```python
from build123d import *

# Parameters (mm, degrees)
F1_DEPTH = 19.05
F2_W     = 6.35
F2_H     = 28.8036865525
F3_DEPTH = 25.4
F4_R     = 5.08
F6_D     = 5.1054


# Not quite as in the source:
# - a feature names something its author has since deleted; it is built from what else it names


with BuildPart() as f1:
    # F0 (on Front) → F1 (new body, symmetric)
    with BuildSketch(Plane.XZ):
        with BuildLine():
            Line((-63.5, 3.175), (-63.5, -3.175))
            Line((-63.5, -3.175), (-25.8909725642, -3.175))
            ThreePointArc((-25.8909725642, -3.175), (-21.6829722848, -1.5805476707), (-19.5881864455, 2.4020917642))
            ThreePointArc((-19.5881864455, 2.4020917642), (0, 19.7349206501), (19.5881864455, 2.4020917642))
            ThreePointArc((19.5881864455, 2.4020917642), (21.6829722848, -1.5805476707), (25.8909725642, -3.175))
            Line((25.8909725642, -3.175), (63.5, -3.175))
            Line((63.5, -3.175), (66.675, -3.175))
            ThreePointArc((66.675, -3.175), (68.9200640303, -2.2450640303), (69.85, 0))
            Line((69.85, 0), (69.85, 27.0641443402))
            ThreePointArc((69.85, 27.0641443402), (70.3149679849, 28.1866763553), (71.4375, 28.6516443402))
            Line((71.4375, 28.6516443402), (87.1900793672, 28.6516443402))
            Line((87.1900793672, 28.6516443402), (87.1900793672, 35.0016443402))
            Line((87.1900793672, 35.0016443402), (66.675, 35.0016443402))
            ThreePointArc((66.675, 35.0016443402), (64.4299359697, 34.0717083704), (63.5, 31.8266443402))
            Line((63.5, 31.8266443402), (63.5, 4.7625))
            ThreePointArc((63.5, 4.7625), (63.0350320151, 3.6399679849), (61.9125, 3.175))
            Line((61.9125, 3.175), (31.0048133776, 3.175))
            ThreePointArc((31.0048133776, 3.175), (27.2311418069, 4.4179555635), (24.9347949838, 7.6602274404))
            ThreePointArc((24.9347949838, 7.6602274404), (0, 26.0849206501), (-24.9347949838, 7.6602274404))
            ThreePointArc((-24.9347949838, 7.6602274404), (-27.2311418069, 4.4179555635), (-31.0048133776, 3.175))
            Line((-31.0048133776, 3.175), (-63.5, 3.175))
        make_face()
    extrude(amount=F1_DEPTH, both=True)

    # F2 (on face) → F3 (cut)
    with BuildSketch(Plane.YZ.offset(87.1900793672)):
        with Locations((0, 20.5998010639)):
            Rectangle(F2_W, F2_H)
    extrude(amount=-F3_DEPTH, mode=Mode.SUBTRACT)

    # F4
    f4_edges = [f1.edges().sort_by_distance(p)[0] for p in [
        (-63.5, -19.05, 0),
        (-63.5, 19.05, 0),
        (87.190079, 19.05, 31.826644),
        (87.190079, 3.175, 31.826644),
        (87.190079, -3.175, 31.826644),
        (87.190079, -19.05, 31.826644),
    ]]
    fillet(f4_edges, radius=F4_R)

    # F6 (through all)
    with Locations(Plane.XY.offset(3.175)):
        with Locations((-54.6063743532, 12.3959155753), (-54.6063743532, -13.8984508812), (52.6370815933, 12.3959155753), (52.0736314356, -13.8984508812)):
            Hole(F6_D / 2)


solid = f1.part
```
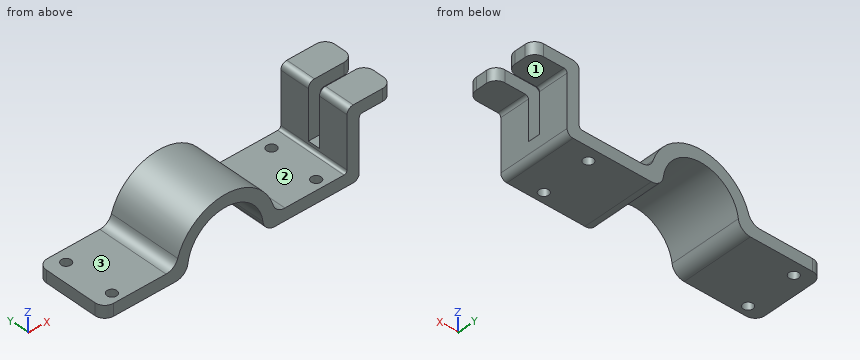
The model under review builds one solid part; all positions refer to its coordinate system, in mm. Face numbers are marked on the shaded views. A direction names the side the tool comes from. Coordinates: 2 decimals unless noted, no trailing zeros. Write each loop counter-clockwise with the first axis right and the second up, starting at its lowest first coordinate (ties: lowest second). Pieces come first, ordered by that corner, then holes. Notation, with made-up numbers: (-31, 11) -> (11, 11) arc R21 ccw to (11, 15) -> close; hole circle Ø1 at (9.5, 70.25). An arc over 180 degrees is marked (long way). One line per item, written item: value. Start each with the question number.
Q1. Add section A-A, the plane x = 73. Give the boundary of the cut face in (y, z) (3 decimals), then the cut area to 3 significant figures.
Q2. To check wall thickness, follow probe 1 along X at (y, z) = (-0.5, 5.5); probe 2 along Y at (x, z) = (66.5, 14.5) (3 decimals); probe 3 along Z at (x, y) = (62, -11) (3 decimals). State the ranges of each line that lie inside material, in increasing order.
Q3. Clearance check with flat-ended pins moving along their axes: P1, Ø8, axis at x = -54.61, y = 12.4, coming from the -Z side (3 decimals); P2, Ø5, axis at x = 68, y = 0, coming from the +Z side; P3, Ø8, axis at y = -7.5, z = 20, coming from the +X side; P4, Ø16, axis at x = -42, y = -5.5, coming from the +Z side (3 decimals). State where each tip first meets the part, or that it passes through.
Q4. For the marked faces 1, 2 and 3, list the 3-axis set-ups (+Z, -Z, +X, -X, +Y, -Y) from which the entire face can be reached by the end or side of a thin tool; tool diameter is ignored.
Q5. Add section B-B, the plane z = 11. Give the boundary of the cut face in (x, y) (3 decimals), then the cut area to 3 significant figures.
Q6. Add section D-D, the plane z = 18. Give the boundary of the cut face in (x, y) (3 decimals), then the cut area to 3 significant figures.
Response:
1. outline: (-19.05, 28.652) -> (-3.175, 28.652) -> (-3.175, 35.002) -> (-19.05, 35.002) -> close; (3.175, 28.652) -> (19.05, 28.652) -> (19.05, 35.002) -> (3.175, 35.002) -> close
1. area: 202 mm²
2. probe 1: -26.09 to -18.95, 18.95 to 26.09, 63.5 to 69.85
2. probe 2: -19.05 to -3.175, 3.175 to 19.05
2. probe 3: -3.175 to 3.177
3. P1: z = -3.175
3. P2: z = 6.2
3. P3: x = 69.85
3. P4: z = 3.175
4. face 1: -Z, +X, +Y, -Y
4. face 2: +Z, +Y, -Y
4. face 3: +Z, -X, +Y, -Y
5. outline: (-23.652, -19.05) -> (-16.385, -19.05) -> (-16.385, 19.05) -> (-23.652, 19.05) -> close; (16.385, -19.05) -> (23.652, -19.05) -> (23.652, 19.05) -> (16.385, 19.05) -> close; (63.5, -19.05) -> (69.85, -19.05) -> (69.85, -3.175) -> (63.5, -3.175) -> close; (63.5, 3.175) -> (69.85, 3.175) -> (69.85, 19.05) -> (63.5, 19.05) -> close
5. area: 755 mm²
6. outline: (-18.879, -19.05) -> (-8.091, -19.05) -> (-8.091, 19.05) -> (-18.879, 19.05) -> close; (8.091, -19.05) -> (18.879, -19.05) -> (18.879, 19.05) -> (8.091, 19.05) -> close; (63.5, -19.05) -> (69.85, -19.05) -> (69.85, -3.175) -> (63.5, -3.175) -> close; (63.5, 3.175) -> (69.85, 3.175) -> (69.85, 19.05) -> (63.5, 19.05) -> close
6. area: 1,020 mm²
